Read the model definition and answer for the solid it produces. Units are mm, in the model's axes. Face numbers are marked on the shaded views. A direction names the side the tool comes from. Give positions to 0.01 mm unless a question says otherwise; leave off trailing zeros. Write each loop counter-clockwise with the first axis right and the second up, starting at its lowest first coordinate (ties: lowest second). Pieces come first, ordered by that corner, then holes.
```python
from build123d import *

# Parameters (mm, degrees)
SKETCH_1_R             = 30
EXTRUDE_1_DEPTH        = 5
SKETCH_2_R             = 20
EXTRUDE_2_DEPTH        = 40
SKETCH_5_R             = 10
EXTRUDE_3_DEPTH        = 71
CUT_EXTRUDE_2_REACH    = 118
SKETCH_6_R             = 5
SKETCH_7_W             = 15
SKETCH_7_H             = 15
CUT_EXTRUDE_3_DEPTH    = 2
SKETCH_8_W             = 15
SKETCH_8_H             = 15
CUT_EXTRUDE_4_DEPTH    = 2
HOLE_WIZARD_M4_2_D     = 3.3
HOLE_WIZARD_M4_2_DEPTH = 5
SKETCH_21_W            = 6
SKETCH_21_H            = 15
CUT_EXTRUDE_5_DEPTH    = 2
SKETCH_22_W            = 15
SKETCH_22_H            = 6
CUT_EXTRUDE_6_DEPTH    = 2


with BuildPart() as part:
    # 스케치1 → 보스-돌출1 (new body)
    with BuildSketch(Plane(origin=(0, 0, 0), x_dir=(1, 0, 0), z_dir=(0, 1, 0))):
        Circle(SKETCH_1_R)
    extrude(amount=EXTRUDE_1_DEPTH)

    # 스케치2 → 보스-돌출2 (add)
    with BuildSketch(Plane(origin=(0, 5, 0), x_dir=(1, 0, 0), z_dir=(0, 1, 0))):
        Circle(SKETCH_2_R)
    extrude(amount=EXTRUDE_2_DEPTH)

    # 스케치5 → 보스-돌출3 (add)
    with BuildSketch(Plane(origin=(0, 45, 0), x_dir=(1, 0, 0), z_dir=(0, 1, 0))):
        Circle(SKETCH_5_R)
    extrude(amount=EXTRUDE_3_DEPTH)

    # 스케치6 → 컷-돌출2 (cut, up to next)
    with BuildSketch(Plane(origin=(0, 116, 0), x_dir=(1, 0, 0), z_dir=(0, 1, 0)), mode=Mode.PRIVATE) as cut_extrude_2_sk1:
        Circle(SKETCH_6_R)
    cut_extrude_2_tool1 = extrude(cut_extrude_2_sk1.sketch, amount=-CUT_EXTRUDE_2_REACH, mode=Mode.PRIVATE) & part.part
    add(cut_extrude_2_tool1.solids().sort_by_distance((0, 116, 0))[0], mode=Mode.SUBTRACT)

    # 스케치7 → 컷-돌출3 (cut)
    with BuildSketch(Plane(origin=(0, 0, -10), x_dir=(-1, 0, 0), z_dir=(0, 0, -1))):
        with Locations((0, 78.5)):
            Rectangle(SKETCH_7_W, SKETCH_7_H)
    extrude(amount=-CUT_EXTRUDE_3_DEPTH, mode=Mode.SUBTRACT)

    # 스케치8 → 컷-돌출4 (cut)
    with BuildSketch(Plane(origin=(-8.660254038, 0, 5), x_dir=(0, -1, 0), z_dir=(-0.866025404, 0, 0.5))):
        with Locations((-78.5, 0)):
            Rectangle(SKETCH_8_W, SKETCH_8_H)
    extrude(amount=-CUT_EXTRUDE_4_DEPTH, mode=Mode.SUBTRACT)

    # M4 나사 구멍2
    with Locations(Plane(origin=(0, 5, 0), x_dir=(1, 0, 0), z_dir=(0, 1, 0))):
        with Locations((0, 25), (21.650635095, 12.5), (21.650635095, -12.5), (-21.650635095, 12.5), (-21.650635095, -12.5), (0, -25)):
            Hole(HOLE_WIZARD_M4_2_D / 2, depth=HOLE_WIZARD_M4_2_DEPTH)

    # 스케치21 → 컷-돌출5 (cut)
    with BuildSketch(Plane(origin=(-8.660254038, 0, 5), x_dir=(0, -1, 0), z_dir=(-0.866025404, 0, 0.5))):
        with Locations((-111, 0)):
            Rectangle(SKETCH_21_W, SKETCH_21_H)
    extrude(amount=-CUT_EXTRUDE_5_DEPTH, mode=Mode.SUBTRACT)

    # 스케치22 → 컷-돌출6 (cut)
    with BuildSketch(Plane(origin=(0, 0, -10), x_dir=(-1, 0, 0), z_dir=(0, 0, -1))):
        with Locations((0.623419069, 111)):
            Rectangle(SKETCH_22_W, SKETCH_22_H)
    extrude(amount=-CUT_EXTRUDE_6_DEPTH, mode=Mode.SUBTRACT)


solid = part.part
```
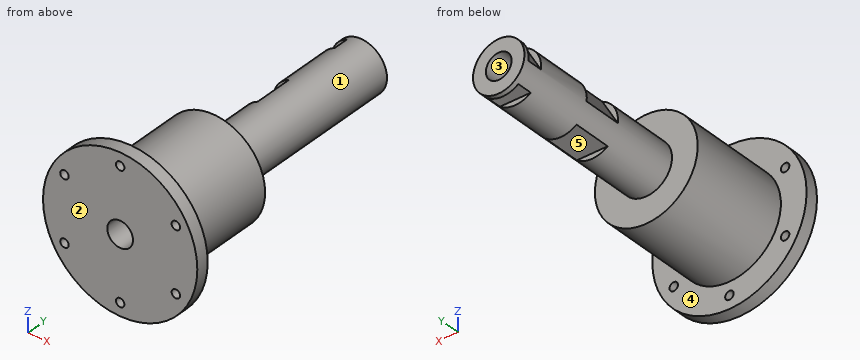
Item 1: Find the intervals of material crossed by line 1 along Z through (x, y) = (0, 2.7); line 2 along X through (y, z) = (1.8, 12.5); line 3 along Z through (x, y) = (0, 64), in increasing order.
Result set:
line 1: z = -30 to -26.65, -23.35 to -5, 5 to 23.35, 26.65 to 30
line 2: x = -27.27 to -23.3, -20 to 20, 23.3 to 27.27
line 3: z = -10 to -5, 5 to 10
Item 2: Determine the mould class of the marked faces 3, 4 and 5 for opening direction Y: pulls with the +Y half, pulls with the -Y half, needs draft (parallel to the pull), parting line crosses it, or undercut.
Result set:
face 3: needs draft
face 4: pulls with the +Y half
face 5: undercut
Item 3: Which of the six approach directions +Z, -Z, +X, -X, +Y, -Y give full straight-line access (tool end or side, diameter ignored) to the marked faces 1 and 2?
Result set:
face 1: +Y
face 2: +Z, -Z, +X, -X, -Y
Item 4: Each of these flat-tipped pins is pushed along its axis until it touches: pin 1 Ø10 at (x, y) = (-14, 24.5) entering from +Z; pin 2 Ø8 at (x, y) = (0, 68) entering from +Z; pin 3 Ø2 at (y, z) = (38.5, -2.5) entering from +X; pin 4 Ø2 at (x, z) = (0, -25) entering from +Y. Where does it stop, or does it pass through?
Result set:
pin 1: stops at z = 17.86
pin 2: stops at z = 10
pin 3: stops at x = 19.94
pin 4: passes through
Item 5: Section C-C (y = 88) is taken. Write down the section's boundary in (x, z).
Result set:
outline: circle Ø20 at (0, 0); hole circle Ø10 at (0, 0)
Item 6: Section D-D (z = -12.5) is taken. Write down the section's boundary in (x, y), and give its area (3 significant figures).
Result set:
outline: (-27.27, 0) - (-23.3, 0) - (-23.3, 5) - (-27.27, 5) - close; (-20, 0) - (20, 0) - (20, 5) - (15.61, 5) - (15.61, 45) - (-15.61, 45) - (-15.61, 5) - (-20, 5) - close; (23.3, 0) - (27.27, 0) - (27.27, 5) - (23.3, 5) - close
area: 1,490 mm2
Item 7: Section A-A (x = 0) is taken. Give the number of separate pieces and of enclosed holes in the cut face, and give its area (4 significant figures).
Result set:
separate pieces: 4
enclosed holes: 0
area: 2,085 mm2
Item 8: Section B-B (z = -25) is taken. Write down the section's boundary in (x, y), and give its area (3 significant figures).
Result set:
outline: (-16.58, 0) - (-1.65, 0) - (-1.65, 5) - (-16.58, 5) - close; (1.65, 0) - (16.58, 0) - (16.58, 5) - (1.65, 5) - close
area: 149 mm2
